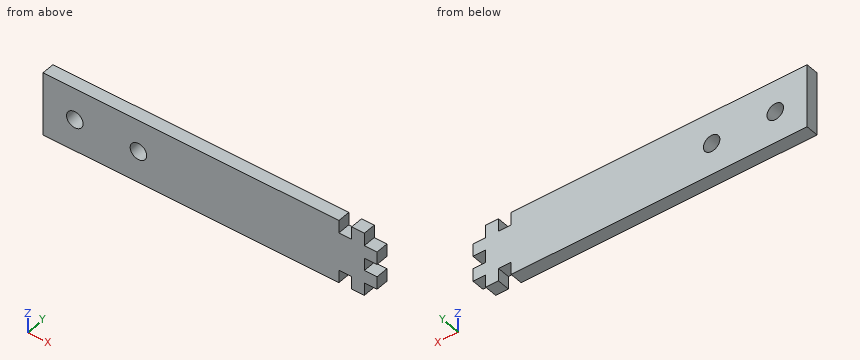
from build123d import *

# Parameters (mm, degrees)
SKETCH1_W               = 66.675
SKETCH1_H               = 12.7
BOSS_EXTRUDE1_DEPTH     = 2.54
CUT_EXTRUDE1_DEPTH      = 1.27
CUT_EXTRUDE1_DEPTH_BACK = 68.921257534
SKETCH3_W               = 2.54
SKETCH3_H               = 2.54
SKETCH4_R               = 1.651
CUT_EXTRUDE2_DEPTH      = 68.921257534
SKETCH5_W               = 2.54
SKETCH5_H               = 2.54
CUT_EXTRUDE3_DEPTH      = 68.921257534


with BuildPart() as part:
    # Sketch1 → Boss-Extrude1 (new body)
    with BuildSketch(Plane(origin=(0, 0, 0), x_dir=(1, 0, 0), z_dir=(0, 1, 0))):
        with Locations((33.3375, 6.35)):
            Rectangle(SKETCH1_W, SKETCH1_H)
    extrude(amount=BOSS_EXTRUDE1_DEPTH)

    # Sketch3 → Cut-Extrude1 (cut, two sides: drawn at the far end of the back side and taken through both)
    with BuildSketch(Plane(origin=(0, 2.54, 0), x_dir=(1, 0, 0), z_dir=(0, 1, 0)).offset(-CUT_EXTRUDE1_DEPTH_BACK)):
        with Locations((65.405, 11.43)):
            Rectangle(SKETCH3_W, SKETCH3_H)
        with Locations((65.405, 1.27)):
            Rectangle(SKETCH3_W, SKETCH3_H)
        with Locations((65.405, 6.35)):
            Rectangle(SKETCH3_W, SKETCH3_H)
    extrude(amount=CUT_EXTRUDE1_DEPTH + CUT_EXTRUDE1_DEPTH_BACK, mode=Mode.SUBTRACT)

    # Sketch4 → Cut-Extrude2 (cut, through all)
    with BuildSketch(Plane(origin=(0, 2.54, 0), x_dir=(1, 0, 0), z_dir=(0, 1, 0))):
        with Locations(Location((6.35, 6.35, 0), (0, 0, 270))):
            Circle(SKETCH4_R)
        with Locations(Location((19.05, 6.35, 0), (0, 0, 270))):
            Circle(SKETCH4_R)
    extrude(amount=-CUT_EXTRUDE2_DEPTH, mode=Mode.SUBTRACT)

    # Sketch5 → Cut-Extrude3 (cut, through all)
    with BuildSketch(Plane(origin=(0, 2.54, 0), x_dir=(1, 0, 0), z_dir=(0, 1, 0))):
        with Locations((60.325, 1.27)):
            Rectangle(SKETCH5_W, SKETCH5_H)
        with Locations((60.325, 11.43)):
            Rectangle(SKETCH5_W, SKETCH5_H)
    extrude(amount=-CUT_EXTRUDE3_DEPTH, mode=Mode.SUBTRACT)


solid = part.part
Design review of the part built by this model. Coordinates are the model's own, in mm. Round coordinates to 2 decimals unless told otherwise and drop trailing zeros. Loops run counter-clockwise (first coordinate to the right, second up) from the corner with the lowest first, then second, coordinate; pieces in that order, holes last. Notation, with made-up numbers: M -33.75,-36 L 1.25,-36 A21 ccw 1.25,-13 Z; hole C 88,87 d9. An arc over 180 degrees is marked long. Answer as a JSON object with one key per item and string values.
Item 1: Wall thickness on L1, parallel to X at y = 0.65, z = -6.35 (3 decimals); L2, parallel to X at y = 2.2, z = -5.5 (3 decimals); L3, parallel to Z at x = 61.5, y = 1.15: over which ranges is each line inside the solid? List them lowest first. Write a range as from..to.
Answer sheet:
{"L1": "x = 0..4.699, 8.001..17.399, 20.701..64.135", "L2": "x = 0..4.935, 7.765..17.635, 20.465..64.135", "L3": "z = -10.16..-2.54"}
Item 2: Clearance check with flat-ended pins moving along their axes: P1, Ø2, axis at x = 6.35, z = -6.35, coming from the -Y side; P2, Ø0.8, axis at y = 1, z = -11, coming from the +X side (3 decimals); P3, Ø1.3, axis at x = 60, y = 1.5, coming from the +Z side. State where each tip first meets the part, or that it passes through.
Answer sheet:
{"P1": "passes through", "P2": "stops at x = 64.135", "P3": "stops at z = -2.54"}
Item 3: We need section C-C on y = 1.75. Give the boundary of the cut face in (x, z) (3 decimals), and give its area (3 significant figures).
Answer sheet:
{"outline": "M 0,-12.7 L 59.055,-12.7 L 59.055,-10.16 L 61.595,-10.16 L 61.595,-12.7 L 64.135,-12.7 L 64.135,-10.16 L 66.675,-10.16 L 66.675,-7.62 L 64.135,-7.62 L 64.135,-5.08 L 66.675,-5.08 L 66.675,-2.54 L 64.135,-2.54 L 64.135,0 L 61.595,0 L 61.595,-2.54 L 59.055,-2.54 L 59.055,0 L 0,0 Z; hole C 6.35,-6.35 d3.302; hole C 19.05,-6.35 d3.302", "area": "797 mm^2"}
Item 4: We need section A-A on x = 6.35. Give the boundary of the cut face in (y, z), and give its area (3 significant figures).
Answer sheet:
{"outline": "M 0,-12.7 L 2.54,-12.7 L 2.54,-8 L 0,-8 Z; M 0,-4.7 L 2.54,-4.7 L 2.54,0 L 0,0 Z", "area": "23.9 mm^2"}
Item 5: We need section B-B on z = -6.35. Give the boundary of the cut face in (x, y) (3 decimals), and give its area (3 significant figures).
Answer sheet:
{"outline": "M 0,0 L 4.699,0 L 4.699,2.54 L 0,2.54 Z; M 8.001,0 L 17.399,0 L 17.399,2.54 L 8.001,2.54 Z; M 20.701,0 L 64.135,0 L 64.135,2.54 L 20.701,2.54 Z", "area": "146 mm^2"}
Item 6: We need section D-D on x = 61. Give the boundary of the cut face in (y, z).
Answer sheet:
{"outline": "M 0,-10.16 L 2.54,-10.16 L 2.54,-2.54 L 0,-2.54 Z"}
